The drawing under review shows one solid part. Ordinate dimensions are in mm from its lowest x, y, z. Give positions to 0.01 mm unless a question says otherwise; leave off trailing zeros. Loops run counter-clockwise (first coordinate to the right, second up) from the corner with the lowest first, then second, coordinate; pieces in that order, holes last. Notation, with made-up numbers: M -0.75,58.25 L 52.25,58.25 A16 ccw 52.25,68.25 Z; hole C -22,34 d10. An arc over 180 degrees is marked long. Write item = value, one per line. Start each with the question number.
1. We need section A-A on z = 3.75. Give the boundary of the cut face in (x, y), then the cut area to 3 significant figures.
2. We need section C-C on y = 31.5. Give the boundary of the cut face in (x, z).
3. We need section B-B on x = 9.5. Give the boundary of the cut face in (y, z).
4. Wall thickness on line 1 along Y through (x, z) = (9.5, 5.5); line 2 along Y through (x, z) = (7.75, 5.25); line 3 along X through (y, z) = (31, 7): over which ranges is each line inside the solid? List them lowest first. Write a range as from..to.
5. Draft analysis for pull direction X (two halves, no side actions). For the marked faces 1, 2 and 3, state which applies: pulls with the +X half, pulls with the -X half, needs draft (parallel to the pull), parting line crosses it, or undercut.
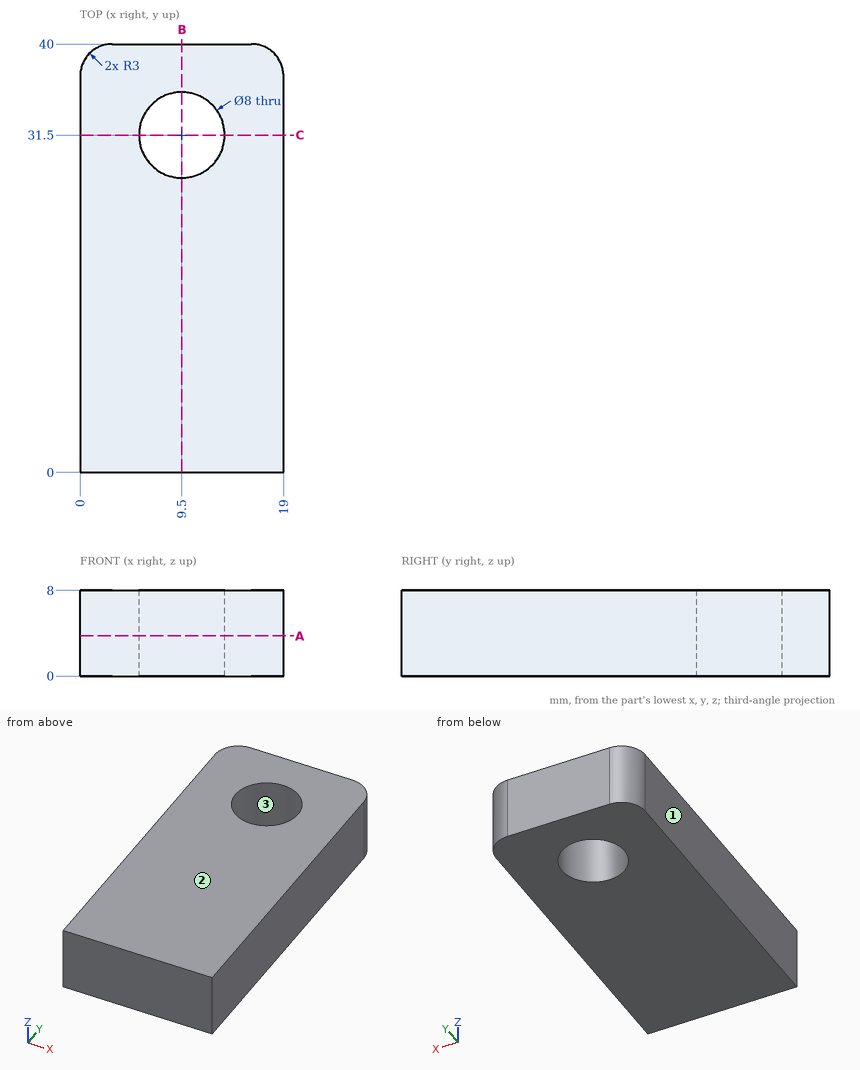
Final values:
q1.outline = M 0,0 L 19,0 L 19,37 A3 ccw 16,40 L 3,40 A3 ccw 0,37 Z; hole C 9.5,31.5 d8
q1.area = 706 mm²
q2.outline = M 0,0 L 5.5,0 L 5.5,8 L 0,8 Z; M 13.5,0 L 19,0 L 19,8 L 13.5,8 Z
q3.outline = M 0,0 L 27.5,0 L 27.5,8 L 0,8 Z; M 35.5,0 L 40,0 L 40,8 L 35.5,8 Z
q4.line_1 = 0..27.5, 35.5..40
q4.line_2 = 0..27.9, 35.1..40
q4.line_3 = 0..5.53, 13.47..19
q5.face_1 = pulls with the -X half
q5.face_2 = needs draft
q5.face_3 = undercut
